Check sheet for the modelled part. Datum: model origin and axes. Units: mm. Face numbers are marked on the shaded views. A direction names the side the tool comes from. Round coordinates to 2 decimals unless told otherwise and drop trailing zeros. Order: outer loops, then holes, each group sorted by start corner. A loop starts at its lowest first (then second) coordinate and runs counter-clockwise, first axis right, second up. Notation, with made-up numbers: (74, -35) -> (89, -35) arc R29 ccw to (89, -4) -> close; hole circle Ø6 at (-36, -17). An arc over 180 degrees is marked (long way). Answer in a Markdown table with one row per item.
```python
from build123d import *

# Parameters (mm, degrees)
SKETCH_1_W               = 400
SKETCH_1_H               = 150
EXTRUDE_1_DEPTH          = 300
SKETCH_2_R               = 30
EXTRUDE_2_DEPTH          = 20
SKETCH_3_R               = 30
EXTRUDE_3_DEPTH          = 20
EXTRUDE_START            = 20
SKETCH_6_R               = 30
EXTRUDE_4_DEPTH          = 20
SKETCH_7_R               = 30
EXTRUDE_5_DEPTH          = 20
SKETCH_8_W               = 200
SKETCH_8_H               = 15
EXTRUDE_6_DEPTH          = 80
SKETCH_9_R               = 20
EXTRUDE_7_DEPTH          = 20
MIRROR_4_COPY_1_SKETCH_R = 20
MIRROR_4_COPY_1_DEPTH    = 20
SKETCH_10_R              = 2
CUT_EXTRUDE_1_DEPTH      = 10


with BuildPart() as part:
    # 草图1 → 凸台-拉伸1 (new body)
    with BuildSketch(Plane.XY):
        Rectangle(SKETCH_1_W, SKETCH_1_H)
    extrude(amount=-EXTRUDE_1_DEPTH)

    # 草图2 → 凸台-拉伸2 (add)
    with BuildSketch(Plane(origin=(200, 0, 0), x_dir=(0, 0, -1), z_dir=(1, 0, 0))):
        with Locations(Location((75, 0, 0), (0, 0, 90))):
            Circle(SKETCH_2_R)
        with Locations(Location((225, 0, 0), (0, 0, 90))):
            Circle(SKETCH_2_R)
    extrude(amount=EXTRUDE_2_DEPTH)

    # 草图3 → 凸台-拉伸3 (add)
    with BuildSketch(Plane(origin=(220, 0, 0), x_dir=(0, 0, -1), z_dir=(1, 0, 0))):
        with Locations(Location((75, 0, 0), (0, 0, 90))):
            Circle(SKETCH_3_R)
    extrude(amount=EXTRUDE_3_DEPTH)

    # 草图6 → 凸台-拉伸4 (add)
    with BuildSketch(Plane.ZY.offset(200).offset(EXTRUDE_START)):
        with Locations(Location((-225, 0, 0), (0, 0, 90))):
            Circle(SKETCH_6_R)
        with Locations(Location((-75, 0, 0), (0, 0, 90))):
            Circle(SKETCH_6_R)
    extrude(amount=-EXTRUDE_4_DEPTH)

    # 草图7 → 凸台-拉伸5 (add)
    with BuildSketch(Plane.ZY.offset(220).offset(EXTRUDE_START)):
        with Locations(Location((-225, 0, 0), (0, 0, 90))):
            Circle(SKETCH_7_R)
    extrude(amount=-EXTRUDE_5_DEPTH)

    # 草图8 → 凸台-拉伸6 (add)
    with BuildSketch(Plane.XY):
        with Locations((0, -47.5)):
            Rectangle(SKETCH_8_W, SKETCH_8_H)
    extrude_6 = extrude(amount=EXTRUDE_6_DEPTH)

    # 镜向2: 凸台-拉伸6 across plane
    add(extrude_6.mirror(Plane.XY.offset(-150)))

    # 草图9 → 凸台-拉伸7 (add)
    with BuildSketch(Plane(origin=(100, 0, 0), x_dir=(0, 0, -1), z_dir=(1, 0, 0))):
        with Locations(Location((-80, -47.5, 0), (0, 0, 337.975687163))):
            Circle(SKETCH_9_R)
    extrude_7 = extrude(amount=EXTRUDE_7_DEPTH)

    # 镜向3: 凸台-拉伸7 across plane
    add(extrude_7.mirror(Plane.XY.offset(-150)))

    # 镜向4: 凸台-拉伸7 across plane
    add(extrude_7.mirror(Plane(origin=(0, 0, 0), x_dir=(0, 0, 1), z_dir=(1, 0, 0))))

    # 镜向4 copy 1 sketch → 镜向4 copy 1 (add)
    with BuildSketch(Plane(origin=(-100, 0, -300), x_dir=(0, 0, 1), z_dir=(-1, 0, 0))):
        with Locations(Location((-80, -47.5, 0), (0, 0, 337.975687163))):
            Circle(MIRROR_4_COPY_1_SKETCH_R)
    extrude(amount=MIRROR_4_COPY_1_DEPTH)

    # 草图10 → 切除-拉伸1 (cut)
    with BuildSketch(Plane(origin=(0, 75, 0), x_dir=(1, 0, 0), z_dir=(0, 1, 0))):
        with Locations(Location((0, 187.5, 0), (0, 0, 270))):
            Circle(SKETCH_10_R)
        with Locations(Location((37.5, 150, 0), (0, 0, 270))):
            Circle(SKETCH_10_R)
        with Locations(Location((0, 112.5, 0), (0, 0, 270))):
            Circle(SKETCH_10_R)
        with Locations(Location((-37.5, 150, 0), (0, 0, 270))):
            Circle(SKETCH_10_R)
    extrude(amount=-CUT_EXTRUDE_1_DEPTH, mode=Mode.SUBTRACT)


solid = part.part
```
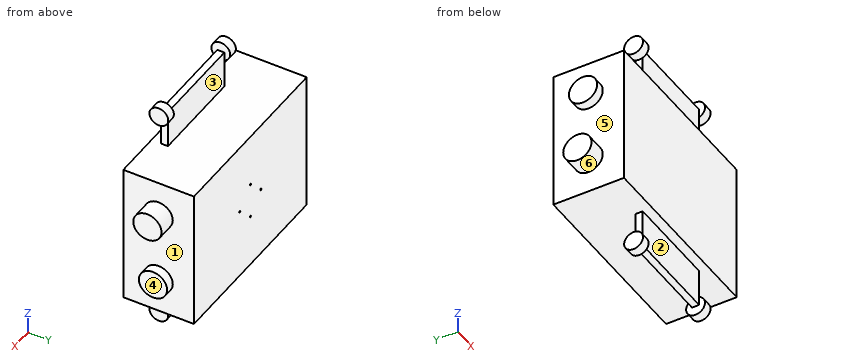
(1) Section check B-B on y = -47.5. Record the boundary of the cut face in (x, z).
Solutions:
| item | result |
|---|---|
| outline | (-200, -300) -> (-100, -300) -> (-100, -360) -> (-120, -360) -> (-120, -400) -> (-100, -400) -> (-100, -380) -> (100, -380) -> (100, -400) -> (120, -400) -> (120, -360) -> (100, -360) -> (100, -300) -> (200, -300) -> (200, 0) -> (100, 0) -> (100, 60) -> (120, 60) -> (120, 100) -> (100, 100) -> (100, 80) -> (-100, 80) -> (-100, 100) -> (-120, 100) -> (-120, 60) -> (-100, 60) -> (-100, 0) -> (-200, 0) -> close |
(2) Section check C-C on x = 209.5. Record the boundary of the cut face in (y, z).
Solutions:
| item | result |
|---|---|
| outline | circle Ø60 at (0, -225); circle Ø60 at (0, -75) |
(3) Draft check along Z on the marked faces 4, 5 and 6. Enter one of: pulls with the +Z half, pulls with the -Z half, needs draft (parallel to the pull), parting line crosses it, or undercut.
Solutions:
| item | result |
|---|---|
| face 4 | needs draft |
| face 5 | undercut |
| face 6 | undercut |
(4) Section check A-A on z = -225. Record the boundary of the cut face in (x, y), plus the area to 3 significant figures.
Solutions:
| item | result |
|---|---|
| outline | (-240, -30) -> (-200, -30) -> (-200, -75) -> (200, -75) -> (200, -30) -> (220, -30) -> (220, 30) -> (200, 30) -> (200, 75) -> (-200, 75) -> (-200, 30) -> (-240, 30) -> close |
| area | 63,600 mm^2 |
(5) Tool access check on the marked faces 1, 2 and 3. Record the directions out of +Z, -Z, +X, -X, +Y, -Y that give a thin tool (end or side, any length) a straight path to the whole face; none if there is none.
Solutions:
| item | result |
|---|---|
| face 1 | +X |
| face 2 | -Z, -Y |
| face 3 | +Z, +Y |
(6) Section check D-D on x = -186.5. Record the boundary of the cut face in (y, z).
Solutions:
| item | result |
|---|---|
| outline | (-75, -300) -> (75, -300) -> (75, 0) -> (-75, 0) -> close |
(7) Scan lines: probe 1 along X at (y, z) = (71, -150); probe 2 along Z at (x, y) = (37, 70); probe 3 along X at (y, z) = (70, -187). Record each from-to range of solid material in increasing order. Write a range as from..to.
Solutions:
| item | result |
|---|---|
| probe 1 | -200..-39.5, -35.5..35.5, 39.5..200 |
| probe 2 | -300..-151.94, -148.06..0 |
| probe 3 | -200..-1.94, 1.94..200 |
(8) Depth check by flat-ended pin: pin 1 Ø6 at (y, z) = (53.5, -75) entering from +X; pin 2 Ø1 at (x, y) = (-158, 0.5) entering from +Z; pin 3 Ø12 at (y, z) = (-51.5, 79.5) entering from -X. Enter the tip coordinate at first touch or a pass-through.
Solutions:
| item | result |
|---|---|
| pin 1 | x = 200 |
| pin 2 | z = 0 |
| pin 3 | x = -120 |
